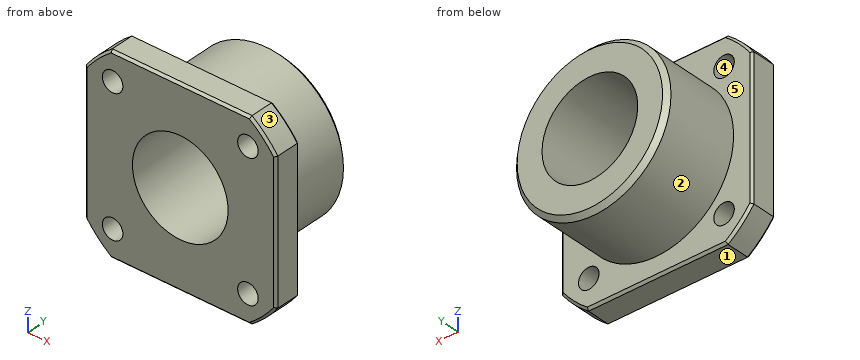
Autodesk Inventor part; units mm, degrees
ref_plane "YZ Plane" through (0, 0, 0) normal (1, 0, 0) x (0, 1, 0)
ref_plane "XZ Plane" through (0, 0, 0) normal (0, 1, 0) x (-1, 0, 0)
ref_plane "XY Plane" through (0, 0, 0) normal (0, 0, 1) x (1, 0, 0)
sketch "Sketch1" plane through (0, 0, 0) normal (0, 1, 0) x (-1, 0, 0)
  line L0 (21, -21) -> (-21, -21)
  line L1 (-21, -21) -> (-21, 21)
  line L2 (-21, 21) -> (21, 21)
  line L3 (21, 21) -> (21, -21)
  point P0 (0, 0)
  dimension "d3" = 42
  dimension "d4" = 42
extrude "Extrusion1" add sketch "Sketch1" along normal blind 6
sketch "Sketch2" plane through (0, 6, 0) normal (0, 1, 0) x (1, 0, 0)
  circle A0 centre (0, 0) radius 16.95
  dimension "d7" = 33.9
extrude "Extrusion2" add sketch "Sketch2" along normal blind 17.1
sketch "Sketch3" plane through (0, 23.1, 0) normal (0, 1, 0) x (1, 0, 0)
  circle A0 centre (0, 0) radius 10.5
  dimension "d10" = 21
extrude "Extrusion3" cut sketch "Sketch3" against normal blind 76.65
sketch "Sketch4" plane through (0, 6, 0) normal (0, 1, 0) x (1, 0, 0)
  point P0 (0, 0)
sketch "Sketch5" plane through (0, 0, 0) normal (0, -1, 0) x (1, 0, 0)
  line L0 (-21, -21) -> (21, -21)
  circle A0 centre (0, 0) radius 10.5
  line L1 (-21, -21) -> (0, 0)
  line L2 (-7.4246, -7.4246) -> (-12.0208, -12.0208)
  line L3 (-12.0208, -12.0208) -> (-17.6777, -17.6777)
  circle A1 centre (-14.8492, -14.8492) radius 4
  circle A2 centre (-14.8492, -14.8492) radius 2.25
  circle A3 centre (14.8492, -14.8492) radius 2.25
  circle A4 centre (14.8492, 14.8492) radius 2.25
  circle A5 centre (-14.8492, 14.8492) radius 2.25
  dimension "d13" = 6.5
  dimension "d14" = 8
  dimension "d15" = 4.5
  dimension "d18" = 360
extrude "Extrusion4" cut sketch "Sketch5" against normal blind 88.15 contours A2 L1 | L1 A2 | A3 | A4 | A5
chamfer "Chamfer1" distance 1 angle 45 1 edges at (-16.95, 23.1, 0)
chamfer "Chamfer2" distance 0.5 angle 45 4 edges at (0, 6, -21) (-21, 6, 0) (0, 6, 21) (21, 6, 0)
sketch "Sketch6" plane through (0, 6, 0) normal (0, 1, 0) x (1, 0, 0)
  line L0 (-20.5, -20.5) -> (-20.5, 20.5)
  circle A0 centre (0, 0) radius 15.95
  line L1 (-20.5, 20.5) -> (0, 0)
  circle A1 centre (0, 0) radius 10.5
  line L2 (-7.4246, 7.4246) -> (-18.3848, 18.3848)
  circle A2 centre (0, 0) radius 26
  circle A3 centre (0, 0) radius 31.7761
  dimension "d28" = 15.5
extrude "Extrusion5" cut sketch "Sketch6" against normal blind 219.6 contours L0 L1 A2 | A3
chamfer "Chamfer3" distance 0.5 angle 45 12 edges at (-18.3848, 6, -18.3848) (18.3848, 6, -18.3848) (18.3848, 6, 18.3848) (-18.3848, 6, 18.3848) (-18.3848, 0, -18.3848) (0, 0, -21) (18.3848, 0, -18.3848) (21, 0, 0) (18.3848, 0, 18.3848) (0, 0, 21) (-18.3848, 0, 18.3848) (-21, 0, 0)
properties part number "608ZZ Ball Screw Support Unit"
The listing builds one solid part. Answer for the finished solid, in the listing's coordinates (mm). Face numbers are marked on the shaded views. A direction names the side the tool comes from. Give positions to 0.01 mm unless a question says otherwise; leave off trailing zeros. Loops run counter-clockwise (first coordinate to the right, second up) from the corner with the lowest first, then second, coordinate; pieces in that order, holes last. Notation, with made-up numbers: (71.5, 34.5) - (80.5, 34.5) arc R13 ccw to (80.5, 44.5) - close; hole circle Ø1 at (78.5, -9.75). An arc over 180 degrees is marked (long way). Answer as a JSON object with one key per item and string values.
1. A cutting plane is placed at C-C (y = 21). Write down the section's boundary in (x, z).
Determined:
{"outline": "circle Ø33.9 at (0, 0); hole circle Ø21 at (0, 0)"}
2. For the marked faces 1 and 2, determine the directions among +Z, -Z, +X, -X, +Y, -Y from which every point of the face is accessible in a straight line to the end or side of a thin tool.
Determined:
{"face 1": "-Z, +X, -X, +Y, -Y", "face 2": "+Y"}
3. A cutting plane is placed at D-D (y = 4). Write down the section's boundary in (x, z), then the cut area to 3 significant figures.
Determined:
{"outline": "(-21, -15.33) arc R26 ccw to (-15.33, -21) - (15.33, -21) arc R26 ccw to (21, -15.33) - (21, 15.33) arc R26 ccw to (15.33, 21) - (-15.33, 21) arc R26 ccw to (-21, 15.33) - close; hole circle Ø4.5 at (-14.85, -14.85); hole circle Ø4.5 at (-14.85, 14.85); hole circle Ø21 at (0, 0); hole circle Ø4.5 at (14.85, -14.85); hole circle Ø4.5 at (14.85, 14.85)", "area": "1,300 mm²"}
4. Find the intervals of material crossed by L1, parallel to X at y = 14.25, z = 0; L2, parallel to X at y = 3.25, z = 14.5; L3, parallel to Z at x = 13.5, y = 5.25, in increasing order. Write a range as [from, to].
Determined:
{"L1": "[-16.95, -10.5], [10.5, 16.95]", "L2": "[-21, -17.07], [-12.63, 12.63], [17.07, 21]", "L3": "[-21, -16.65], [-13.05, 13.05], [16.65, 21]"}
5. Flat-ended cylindrical pins translate along their axes: pin 1 Ø2.5 at (x, z) = (14.85, 14.85) entering from -Y; pin 2 Ø5 at (y, z) = (9, 11) entering from -X; pin 3 Ø4 at (y, z) = (13.5, -12) entering from -X; pin 4 Ø5 at (x, z) = (-14.85, 14.85) entering from +Y. Find the tip coordinate at first contact, or state that the pin passes through.
Determined:
{"pin 1": "through", "pin 2": "x = -14.66", "pin 3": "x = -13.69", "pin 4": "y = 6"}
6. For a pull along Z with two mould halves and no side action, classify the marked faces 3, 4 and 5 as pulls with the +Z half, pulls with the -Z half, needs draft (parallel to the pull), parting line crosses it, or undercut.
Determined:
{"face 3": "pulls with the +Z half", "face 4": "undercut", "face 5": "needs draft"}
7. A cutting plane is placed at B-B (x = 0). Write down the section's boundary in (y, z), then the cut area to 3 significant figures.
Determined:
{"outline": "(0, -20.5) - (0.5, -21) - (5.5, -21) - (6, -20.5) - (6, -16.95) - (22.1, -16.95) - (23.1, -15.95) - (23.1, -10.5) - (0, -10.5) - close; (0, 10.5) - (23.1, 10.5) - (23.1, 15.95) - (22.1, 16.95) - (6, 16.95) - (6, 20.5) - (5.5, 21) - (0.5, 21) - (0, 20.5) - close", "area": "345 mm²"}
8. A cutting plane is placed at A-A (z = 0). Write down the section's boundary in (x, y).
Determined:
{"outline": "(-21, 0.5) - (-20.5, 0) - (-10.5, 0) - (-10.5, 23.1) - (-15.95, 23.1) - (-16.95, 22.1) - (-16.95, 6) - (-20.5, 6) - (-21, 5.5) - close; (10.5, 0) - (20.5, 0) - (21, 0.5) - (21, 5.5) - (20.5, 6) - (16.95, 6) - (16.95, 22.1) - (15.95, 23.1) - (10.5, 23.1) - close"}
